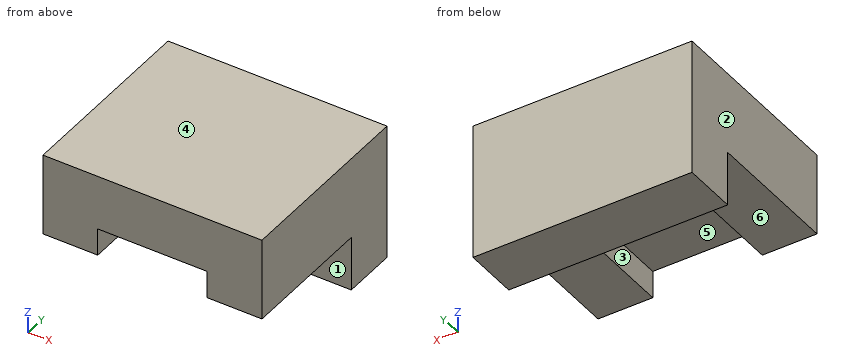
from build123d import *

# Parameters (mm, degrees)
F0_W     = 203.2
F0_H     = 127
F1_DEPTH = 50.8
F2_W     = 203.2
F2_H     = 76.2
F3_DEPTH = 25.4
F5_DEPTH = 101.6


with BuildPart() as f1:
    # F0 (on Front) → F1 (new body)
    with BuildSketch(Plane.XZ):
        with Locations((-26.285635, 11.66383)):
            Rectangle(F0_W, F0_H)
    extrude(amount=F1_DEPTH)

    # F2 (on face) → F3 (join)
    with BuildSketch(Plane.XZ.offset(50.8)):
        with Locations((-26.285635, 37.06383)):
            Rectangle(F2_W, F2_H)
    extrude(amount=F3_DEPTH)

    # F4 (on face) → F5 (join)
    with BuildSketch(Plane.XZ.offset(76.2)):
        Polygon((-77.085635, 24.36383), (24.514365, 24.36383), (24.514365, -1.03617), (75.314365, -1.03617), (75.314365, 75.16383), (-127.885635, 75.16383), (-127.885635, -1.03617), (-77.085635, -1.03617), align=None)
    extrude(amount=F5_DEPTH)


solid = f1.part
Verification items for the finished model (mm, model axes). Face numbers are marked on the shaded views. A direction names the side the tool comes from. Coordinates: 2 decimals unless noted, no trailing zeros. Loops run counter-clockwise (first coordinate to the right, second up) from the corner with the lowest first, then second, coordinate; pieces in that order, holes last. Notation, with made-up numbers: (-7, 68.25) -> (27, 68.25) arc R22 ccw to (27, 107.25) -> close; hole circle Ø10 at (80, 65). An arc over 180 degrees is marked (long way). Answer as CSV lines item,"result".
1) Depth check by flat-ended pin: pin 1 (2 mm diameter, centred on x = -84.5, y = -99, fed in from -Z); pin 2 (12.5 mm diameter, centred on x = -31, z = 7, fed in from -Y). Enter the tip coordinate at first touch or a pass-through.
Found:
pin 1,"stops at z = -1.04"
pin 2,"stops at y = -76.2"
2) Cross-section at A-A, the plane y = -146.5. Record the cut outline in (x, z), then the cut area to 3 significant figures.
Found:
outline,"(-127.89, -1.04) -> (-77.09, -1.04) -> (-77.09, 24.36) -> (24.51, 24.36) -> (24.51, -1.04) -> (75.31, -1.04) -> (75.31, 75.16) -> (-127.89, 75.16) -> close"
area,"12,900 mm2"
3) Cross-section at C-C, the plane z = -5.5. Record the cut outline in (x, y).
Found:
outline,"(-127.89, -50.8) -> (75.31, -50.8) -> (75.31, 0) -> (-127.89, 0) -> close"
4) Tool access check on the marked faces 4, 5 and 6. Record the directions out of +Z, -Z, +X, -X, +Y, -Y that give a thin tool (end or side, any length) a straight path to the whole face; none if there is none.
Found:
face 4,"+Z, +X, -X, +Y, -Y"
face 5,"-Z, -Y"
face 6,"-Z, +X, -X, -Y"
5) Release check for a two-part mould opening along X. For the marked faces 1, 2 and 3 record: +X half, -X half, draft (parallel to the pull), parting line (faces both ways), or undercut.
Found:
face 1,"draft"
face 2,"-X half"
face 3,"undercut"
6) Cross-section at D-D, the plane x = -58.5. Record the cut outline in (y, z).
Found:
outline,"(-177.8, 24.36) -> (-76.2, 24.36) -> (-76.2, -1.04) -> (-50.8, -1.04) -> (-50.8, -51.84) -> (0, -51.84) -> (0, 75.16) -> (-177.8, 75.16) -> close"
7) Cross-section at B-B, the plane x = -80.5. Record the cut outline in (y, z), then the cut area to 3 significant figures.
Found:
outline,"(-177.8, -1.04) -> (-50.8, -1.04) -> (-50.8, -51.84) -> (0, -51.84) -> (0, 75.16) -> (-177.8, 75.16) -> close"
area,"16,100 mm2"
8) Thickness scan on L1, parallel to Z at x = -15, y = -84; L2, parallel to Y at x = -52, z = 15.5; L3, parallel to Y at x = -113, z = -45. Record the ranges inside material, lowest first. Write a range as from..to.
Found:
L1,"z = 24.36..75.16"
L2,"y = -76.2..0"
L3,"y = -50.8..0"
